Could you check a few things on this model? Use its own coordinates, in mm. Face numbers are marked on the shaded views. A direction names the side the tool comes from. Coordinates: 2 decimals unless noted, no trailing zeros. Write each loop counter-clockwise with the first axis right and the second up, starting at its lowest first coordinate (ties: lowest second). Pieces come first, ordered by that corner, then holes.
Item 1: I want a section at B-B on y = 5.5. Please give me the cut outline in (x, z) (3 decimals), then the cut area to 3 significant figures.
Item 2: I want a section at A-A on z = -28. Please give me the cut outline in (x, y), then the cut area to 3 significant figures.
Item 3: If I drill on probe 1 along X at (y, z) = (0.75, -31); probe 2 along Z at (x, y) = (180.5, 2); probe 3 along X at (y, z) = (2, 81.5), over which ranges is the centre line in solid material (lowest first)?
Item 4: I want a section at C-C on x = 22.5. Please give me the cut outline in (y, z), then the cut area to 3 significant figures.
Item 5: For P1, Ø1, axis at x = 53, y = 3, coming from the +Z side; P2, Ø1.6, axis at x = 12.5, y = 5.5, coming from the -Z side; P3, Ø1, axis at x = 26.5, z = 75.5, coming from the +Y side; P4, Ø19.5, axis at x = 12, z = 23, coming from the +Y side, each with a flat end and sliding along its axis, tell me the tip position at first contact or that it passes through.
Item 6: Thinking about a two-plate mould opening in Z: for the marked faces 3 and 4, which applies, +Z half, -Z half, draft (parallel to the pull), parting line (faces both ways), or undercut?
Item 7: I want a section at D-D on x = 89.5. Please give me the cut outline in (y, z), then the cut area to 3 significant figures.
Item 8: Which directions (+Z, -Z, +X, -X, +Y, -Y) give clear straight access to the entire face, cutting with the end or side of a thin tool? Please do the marked faces 1 and 2.
from build123d import *

# Parameters (mm, degrees)
SKETCH1_R           = 3.302
BOSS_EXTRUDE1_DEPTH = 7.112
SKETCH2_W           = 50.8
SKETCH2_H           = 152.4
CUT_EXTRUDE1_DEPTH  = 3.175
SKETCH3_R           = 3.81
BOSS_EXTRUDE2_DEPTH = 7.112
FILLET1_R           = 2.54


with BuildPart() as part:
    # Sketch1 → Boss-Extrude1 (new body)
    with BuildSketch(Plane(origin=(0, 0, 0), x_dir=(1, 0, 0), z_dir=(0, 1, 0))):
        with BuildLine():
            Line((25.4, 85.725), (25.4, -85.725))
            ThreePointArc((25.4, -85.725), (0, -111.125), (-25.4, -85.725))
            Line((-25.4, -85.725), (-25.4, 85.725))
            ThreePointArc((-25.4, 85.725), (0, 111.125), (25.4, 85.725))
        make_face()
        with Locations(Location((0, 85.725, 0), (0, 0, 270))):
            Circle(SKETCH1_R, mode=Mode.SUBTRACT)
        with Locations(Location((0, -85.725, 0), (0, 0, 270))):
            Circle(SKETCH1_R, mode=Mode.SUBTRACT)
        with BuildLine():
            Line((3.302, 73.025), (3.302, -73.025))
            ThreePointArc((3.302, -73.025), (0, -76.327), (-3.302, -73.025))
            Line((-3.302, -73.025), (-3.302, 73.025))
            ThreePointArc((-3.302, 73.025), (0, 76.327), (3.302, 73.025))
        make_face(mode=Mode.SUBTRACT)
    extrude(amount=BOSS_EXTRUDE1_DEPTH)

    # Sketch2 → Cut-Extrude1 (cut)
    with BuildSketch(Plane(origin=(0, 7.112, 0), x_dir=(1, 0, 0), z_dir=(0, 1, 0))):
        Rectangle(SKETCH2_W, SKETCH2_H)
    extrude(amount=-CUT_EXTRUDE1_DEPTH, mode=Mode.SUBTRACT)

    # Sketch3 → Boss-Extrude2 (add)
    with BuildSketch(Plane(origin=(0, 0, 0), x_dir=(1, 0, 0), z_dir=(0, 1, 0))):
        with BuildLine():
            Line((-9.525, 85.725), (-9.525, 133.35))
            Line((-9.525, 133.35), (185.274739587, 133.35))
            ThreePointArc((185.274739587, 133.35), (206.375, 123.825), (185.274739587, 114.3))
            Line((185.274739587, 114.3), (9.525, 114.3))
            Line((9.525, 114.3), (9.525, 85.725))
            Line((9.525, 85.725), (0, 95.25))
            Line((0, 95.25), (-9.525, 85.725))
        make_face()
        with Locations(Location((193.675, 123.825, 0), (0, 0, 270))):
            Circle(SKETCH3_R, mode=Mode.SUBTRACT)
    extrude(amount=BOSS_EXTRUDE2_DEPTH)

    # Fillet1
    fillet1_edges = [part.edges().sort_by_distance(p)[0] for p in [
        (-9.525, 3.556, -133.35),
        (9.525, 3.556, -114.3),
    ]]
    fillet(fillet1_edges, radius=FILLET1_R)


solid = part.part
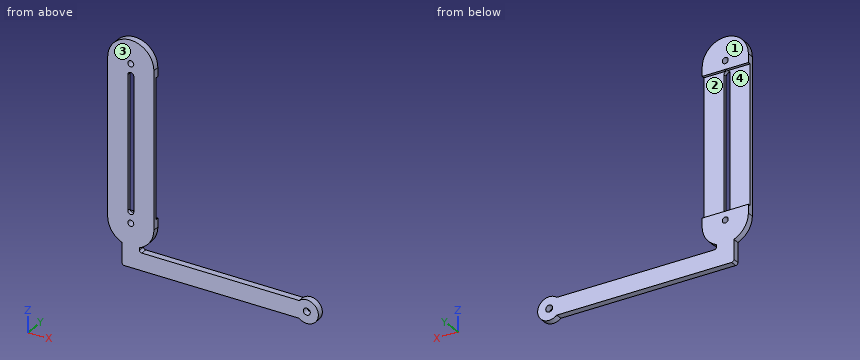
Response values:
1. outline: (-25.4, -85.725) arc R25.4 ccw to (-9.525, -109.271) - (-9.525, -130.81) arc R2.54 ccw to (-6.985, -133.35) - (185.275, -133.35) arc R12.7 ccw (long way) to (185.275, -114.3) - (12.065, -114.3) arc R2.54 cw to (9.525, -111.76) - (9.525, -109.271) arc R25.4 ccw to (25.4, -85.725) - (25.4, -76.2) - (0.907, -76.2) arc R3.302 cw to (-0.907, -76.2) - (-25.4, -76.2) - close; (-25.4, 76.2) - (-0.907, 76.2) arc R3.302 cw to (0.907, 76.2) - (25.4, 76.2) - (25.4, 85.725) arc R25.4 ccw to (-25.4, 85.725) - close; hole circle Ø6.604 at (0, -85.725); hole circle Ø6.604 at (0, 85.725); hole circle Ø7.62 at (193.675, -123.825)
1. area: 7,110 mm2
2. outline: (-25.4, 0) - (-3.3, 0) - (-3.3, 3.94) - (-25.4, 3.94) - close; (3.3, 0) - (25.4, 0) - (25.4, 3.94) - (3.3, 3.94) - close
2. area: 174 mm2
3. probe 1: x = -25.4 to -3.3, 3.3 to 25.4
3. probe 2: z = -133.35 to -114.3
3. probe 3: x = -25.4 to 25.4
4. outline: (0, -133.35) - (7.11, -133.35) - (7.11, -114.3) - (0, -114.3) - close; (0, -97.51) - (7.11, -97.51) - (7.11, -76.2) - (3.94, -76.2) - (3.94, 76.2) - (7.11, 76.2) - (7.11, 97.51) - (0, 97.51) - close
4. area: 1,040 mm2
5. P1: stops at z = -114.3
5. P2: stops at z = -133.35
5. P3: passes through
5. P4: stops at y = 3.94
6. face 3: draft
6. face 4: undercut
7. outline: (0, -133.35) - (7.11, -133.35) - (7.11, -114.3) - (0, -114.3) - close
7. area: 135 mm2
8. face 1: +Z, -Z, +X, -X, +Y
8. face 2: +X, -X, +Y
